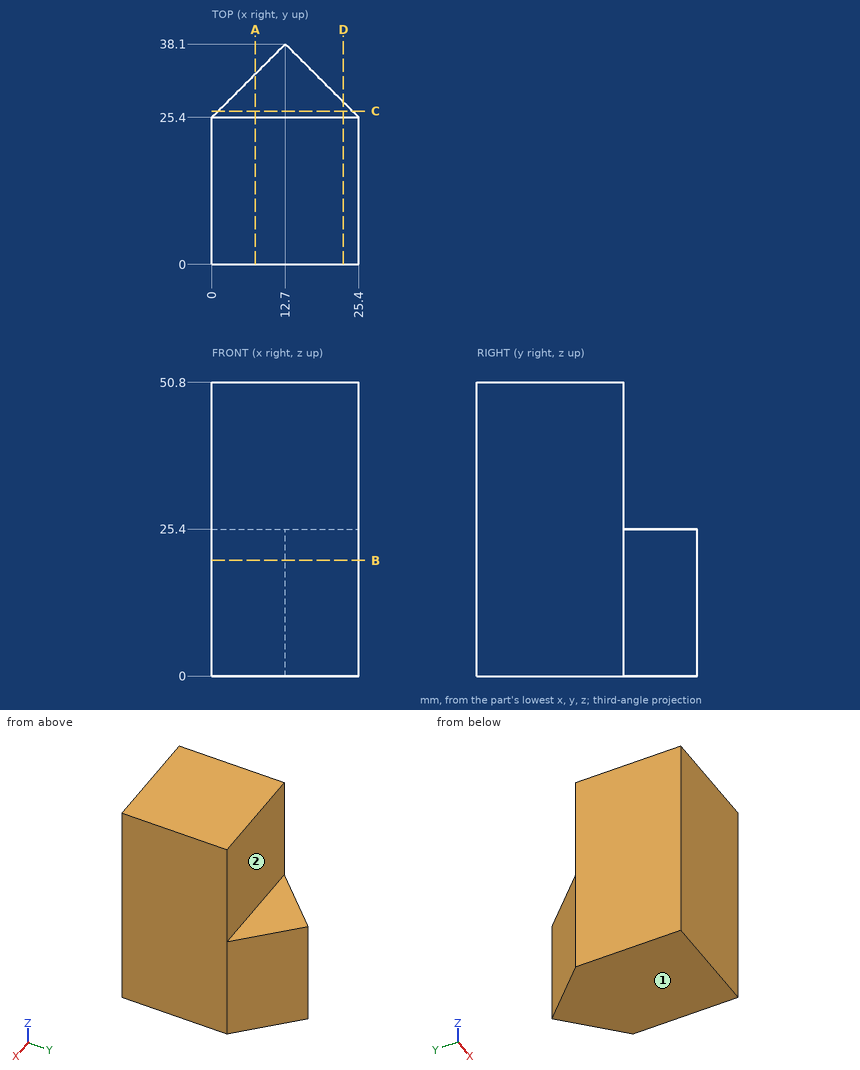
For this review, use the dimensioned drawing (mm, ordinates from the lowest corner) and the shaded views. A direction names the side the tool comes from. Coordinates: 2 decimals unless noted, no trailing zeros. Loops run counter-clockwise (first coordinate to the right, second up) from the corner with the lowest first, then second, coordinate; pieces in that order, holes last. Notation, with made-up numbers: (-38.5, -18) -> (9.5, -18) arc R14 ccw to (9.5, -8) -> close; hole circle Ø6 at (-2.75, 14.5). An arc over 180 degrees is marked (long way). Use a Markdown table: item, result. Add a question column.
1. Machinability: for the marked faces 1 and 2, which of the approach directions +Z, -Z, +X, -X, +Y, -Y give a long, thin tool a straight path to every point of the face, cutting with its end or side? Answer none if there is none.
2. Clearance check with flat-ended pins moving along their axes: pin 1 Ø1.5 at (x, z) = (11, 25.5) entering from +Y; pin 2 Ø6 at (y, z) = (33, 10.5) entering from -X; pin 3 Ø1.5 at (x, z) = (21, 17) entering from +Y. State where each tip first meets the part, or that it passes through.
3. Add section A-A on x = 7.5. Write out the cut boundary in (y, z).
4. Add section C-C on y = 26.5. Write out the cut boundary in (x, z).
5. Add section B-B on z = 20. Write out the cut boundary in (x, y), plus the area to 3 significant figures.
6. Add section D-D on x = 22.75. Write out the cut boundary in (y, z), plus the area to 3 significant figures.
7. To check wall thickness, follow line 1 (Y direction, x = 20.5, z = 26); line 2 (Y direction, x = 8.5, z = 7.5). State the ranges of each line that lie inside material, in increasing order.
Returned:
| question | item | result |
|---|---|---|
| 1 | face 1 | -Z, +X, -X, +Y, -Y |
| 1 | face 2 | +Z, +X, -X, +Y |
| 2 | pin 1 | stops at y = 37.14 |
| 2 | pin 2 | stops at x = 4.6 |
| 2 | pin 3 | stops at y = 30.55 |
| 3 | outline | (0, 0) -> (32.9, 0) -> (32.9, 25.4) -> (25.4, 25.4) -> (25.4, 50.8) -> (0, 50.8) -> close |
| 4 | outline | (1.1, 0) -> (24.3, 0) -> (24.3, 25.4) -> (1.1, 25.4) -> close |
| 5 | outline | (0, 0) -> (25.4, 0) -> (25.4, 25.4) -> (12.7, 38.1) -> (0, 25.4) -> close |
| 5 | area | 806 mm² |
| 6 | outline | (0, 0) -> (28.05, 0) -> (28.05, 25.4) -> (25.4, 25.4) -> (25.4, 50.8) -> (0, 50.8) -> close |
| 6 | area | 1,360 mm² |
| 7 | line 1 | y = 0 to 25.4 |
| 7 | line 2 | y = 0 to 33.9 |
